Read the model definition and answer for the solid it produces. Units are mm, in the model's axes. A direction names the side the tool comes from. Give positions to 0.01 mm unless a question says otherwise; leave off trailing zeros. Loops run counter-clockwise (first coordinate to the right, second up) from the corner with the lowest first, then second, coordinate; pieces in that order, holes last. Notation, with made-up numbers: (89.25, -4) - (136.25, -4) arc R25 ccw to (136.25, 15) - close; hole circle Ø3 at (-2.5, -39.75). An arc over 180 degrees is marked (long way). Put each result on its own line as item: value. Start each with the question number.
1. Given pin 1 Ø1 at (x, y) = (54, -30) entering from -Z; pin 2 Ø4.5 at (y, z) = (-80, 49) entering from -X; pin 3 Ø10 at (x, z) = (-8, -170.5) entering from +Y, each flat-ended and moving along its own axis, determine where each tip first touches the part or whether it passes through.
2. A cutting plane is placed at B-B, the plane y = -13. Determine the outline of the cut face in (x, z).
3. For a pull along Z with two mould halves and no side action, classify faces 5 (the flat face through (-9, -5, -177.8)), 6 (the flat face through (-8.44, -84.39, 49.87)), 7 (the flat face through (-90.819, -80, 49)), 8 (the flat face through (-8.441, -76.187, 48.533)) as released by +Z, released by -Z, zero draft, split by the parting line, or undercut.
4. A cutting plane is placed at C-C, the plane z = -26. Determine the outline of the cut face in (x, y).
5. For faces 1 (the flat face through (41.8, 7.13, 43.87)), 2 (the flat face through (-9, -61.294, -81)), 3 (the flat face through (-9, 66.102, -171)), 4 (the flat face through (84.789, 27, 41)), determine the directions among +Z, -Z, +X, -X, +Y, -Y from which every point of the face is accessible in a straight line to the end or side of a thin tool.
6. A cutting plane is placed at D-D, the plane x = -102.5. Determine the outline of the cut face in (y, z), plus the area to 3 significant figures.
7. Consider L1, parallel to Y at x = 29, z = -23.5; L2, parallel to X at y = 1.5, z = -78; L3, parallel to Z at x = 50, y = 66. Determine where each line is inside the solid, lowest interval first. Write a range as from..to.
8. A cutting plane is placed at A-A, the plane x = 68. Determine the outline of the cut face in (y, z), plus the area to 3 significant figures.
```python
from build123d import *

# Parameters (mm, degrees)
F0_W      = 254
F0_H      = 228.6
F1_DEPTH  = 50.8
F2_W      = 101.6
F2_H      = 115.2657791972
F3_DEPTH  = 165.1
F5_DEPTH  = 279.4
F6_W      = 118.5094341636
F6_H      = 139.5258828998
F7_DEPTH  = 12.7
F8_W      = 167.0939251781
F8_H      = 8.3109661937
F9_DEPTH  = 7.62
F10_W     = 84.7886428237
F10_H     = 39.9433299899
F11_DEPTH = 25.4


with BuildPart() as f1:
    # F0 (on Top) → F1 (new body)
    with BuildSketch(Plane.XY):
        with Locations((-8.4815638786, 0.7548034191)):
            Rectangle(F0_W, F0_H)
    extrude(amount=F1_DEPTH)

    # F2 (on face) → F3 (join)
    with BuildSketch(Plane(origin=(0, 0, 0), x_dir=(1, 0, 0), z_dir=(0, 0, -1))):
        with Locations((-8.3371599585, 3.6606378853)):
            Rectangle(F2_W, F2_H)
    extrude(amount=F3_DEPTH)

    # F4 (on face) → F5 (cut)
    with BuildSketch(Plane.YZ.offset(118.5184361214)):
        Polygon((115.0548034191, 50.8), (-113.5451965809, 50.8), (115.0548034191, 13.6371413246), align=None)
    extrude(amount=-F5_DEPTH, mode=Mode.SUBTRACT)

    # F6 (on face) → F7 (join)
    with BuildSketch(Plane(origin=(0, 0, -165.1), x_dir=(1, 0, 0), z_dir=(0, 0, -1))):
        with Locations((-8.6290575564, 3.6606378853)):
            Rectangle(F6_W, F6_H)
    extrude(amount=F7_DEPTH)

    # F8 (on face) → F9 (join)
    with BuildSketch(Plane(origin=(0, 5.1222588583, 31.5085657224), x_dir=(1, 0, 0), z_dir=(0, 0.1604606782, 0.9870422335))):
        with Locations((-7.2715543211, -87.1428288519)):
            Rectangle(F8_W, F8_H)
    extrude(amount=F9_DEPTH)

    # F10 (on face) → F11 (join)
    with BuildSketch(Plane(origin=(0, 5.1222588583, 31.5085657224), x_dir=(1, 0, 0), z_dir=(0, 0.1604606782, 0.9870422335))):
        with Locations((42.3943214118, 19.971664995)):
            Rectangle(F10_W, F10_H)
    extrude(amount=F11_DEPTH)


solid = f1.part
```
Return value:
1. pin 1: stops at z = 0
1. pin 2: stops at x = -90.82
1. pin 3: stops at y = 66.1
2. outline: (-135.48, 0) - (-59.14, 0) - (-59.14, -165.1) - (-67.88, -165.1) - (-67.88, -177.8) - (50.63, -177.8) - (50.63, -165.1) - (42.46, -165.1) - (42.46, 0) - (118.52, 0) - (118.52, 34.45) - (-135.48, 34.45) - close
3. face 5: released by -Z
3. face 6: released by +Z
3. face 7: zero draft
3. face 8: undercut
4. outline: (-59.14, -61.29) - (42.46, -61.29) - (42.46, 53.97) - (-59.14, 53.97) - close
5. face 1: +Z, +X, -X
5. face 2: +X, -X, -Y
5. face 3: -Z, +X, -X, +Y
5. face 4: +Z, +X, +Y
6. outline: (-113.55, 0) - (115.05, 0) - (115.05, 13.64) - (-113.55, 50.8) - close
6. area: 7,370 mm2
7. L1: y = -61.29..53.97
7. L2: x = -59.14..42.46
7. L3: z = -177.8..-165.1, 0..21.61
8. outline: (-113.55, 0) - (115.05, 0) - (115.05, 13.64) - (44.55, 25.1) - (48.62, 50.17) - (9.2, 56.58) - (5.12, 31.51) - (-76.79, 44.82) - (-75.57, 52.35) - (-83.77, 53.68) - (-84.99, 46.16) - (-113.55, 50.8) - close
8. area: 8,440 mm2
